Autodesk Inventor part; units mm, degrees
ref_plane "YZ Plane" through (0, 0, 0) normal (1, 0, 0) x (0, 1, 0)
ref_plane "XZ Plane" through (0, 0, 0) normal (0, 1, 0) x (-1, 0, 0)
ref_plane "XY Plane" through (0, 0, 0) normal (0, 0, 1) x (1, 0, 0)
sketch "Sketch5" plane through (0, 0, 0) normal (0, 0, 1) x (1, 0, 0)
  line L0 (0, 0) -> (6.35, 0)
  line L1 (6.35, 0) -> (6.35, 25.4)
  line L2 (6.35, 25.4) -> (0, 25.4)
  line L3 (0, 25.4) -> (0, 0)
  dimension "d21" = 25.4
  dimension "d22" = 6.35
extrude "Extrusion3" add sketch "Sketch5" against normal mid plane 38.1
sketch "Sketch6" plane through (0, 0, 0) normal (0, 0, 1) x (1, 0, 0)
  line L0 (6.35, 25.4) -> (6.35, 0)
  line L1 (0, 25.4) -> (6.35, 25.4)
  line L2 (6.35, 0) -> (0, 0)
  line L3 (0, 0) -> (0, 25.4)
  line L4 (6.35, 0) -> (70.8025, 37.2117)
  line L5 (6.35, 0) -> (80.7733, 0) construction
  line L6 (70.8025, 62.6117) -> (70.8025, 37.2117)
  arc A0 (38.9766, 44.237) -> (62.6234, 57.8895) centre (50.8, 51.0632) ccw
  line L7 (6.35, 25.4) -> (38.9766, 44.237)
  line L8 (62.6234, 57.8895) -> (70.8025, 62.6117)
  dimension "d25" = 30
  dimension "d26" = 27.305
  dimension "d29" = 6.35
  dimension "d30" = 50.8
  dimension "d33" = 0
extrude "Extrusion4" add sketch "Sketch6" along normal mid plane 6.35 contours L7 A0 L8 L6 L4 L0
sketch "Sketch7" plane through (6.35, 0, 19.05) normal (1, 0, 0) x (0, 0, -1)
  line L0 (38.1, 25.4) -> (0, 25.4) construction
  line L1 (6.35, 25.4) -> (6.35, 0) construction
  line L2 (31.75, 25.4) -> (31.75, 0) construction
  line L3 (0, 0) -> (0, 25.4) construction
  line L4 (38.1, 25.4) -> (38.1, 0) construction
  line L5 (0, 0) -> (15.875, 0)
  line L6 (22.225, 0) -> (38.1, 0)
  point P0 (19.05, 0)
  point P1 (6.35, 12.7)
  point P2 (31.75, 12.7)
  dimension "d34" = 6.35
  dimension "d35" = 6.35
sketch "Sketch8" plane through (0, 0, 0) normal (0, 0, 1) x (1, 0, 0)
  line L0 (0, 0) -> (0, 25.4)
  line L1 (6.35, 0) -> (0, 0)
  line L2 (70.8025, 37.2117) -> (6.35, 0)
  line L3 (0, 0) -> (6.35, 0)
  line L4 (0, -3.6662) -> (6.35, 0)
  line L5 (0, 0) -> (0, -3.6662)
extrude "Extrusion5" add sketch "Sketch8" along normal mid plane 38.1
hole "Hole3" at (6.35, 12.7, 12.7) at (6.35, 12.7, -12.7) direction (-1, 0, 0) diameter 3.81 end through all countersink diameter 7.0866 countersink angle 82
sketch "Sketch9" plane through (0, 0, 0) normal (0, 0, 1) x (1, 0, 0)
  line L0 (0, -3.6662) -> (0, 25.4)
  line L1 (0, 25.4) -> (6.35, 25.4)
  line L2 (6.35, 25.4) -> (6.35, 0)
  line L3 (6.35, 25.4) -> (38.9766, 44.237)
  line L4 (6.35, 25.4) -> (0, 25.4)
  line L5 (6.35, 25.4) -> (0, 21.7338)
  line L6 (0, 25.4) -> (0, 21.7338)
  point P0 (0, 0)
extrude "Extrusion6" cut sketch "Sketch9" against normal mid plane 38.1
equation "\"d21\" = supportHeight"
equation "\"d22\" = supportWidth"
equation "\"d23\" = totalScrewHoldWidth"
equation "\"d25\" = supportAngle"
equation "\"d26\" = pipeDiameter"
equation "\"d30\" = distanceFromWallToPipeCenter"
equation "\"d31\" = supportWidth"
equation "\"d47\" = totalScrewHoldWidth"
equation "\"d63\" = totalScrewHoldWidth"
equation "\"pipeDiameter\" = 27.305"
equation "\"distanceFromWallToPipeCenter\" = 50.8"
equation "\"supportHeight\" = 25.4"
equation "\"supportWidth\" = 6.35"
equation "\"screwHoldDepth\" = 6.35"
equation "\"totalScrewHoldWidth\" = 38.1"
equation "\"screwPositionFromTop\" = 6.35"
equation "\"supportAngle\" = 30deg"
properties part number "PipeSupport-2_00-030"
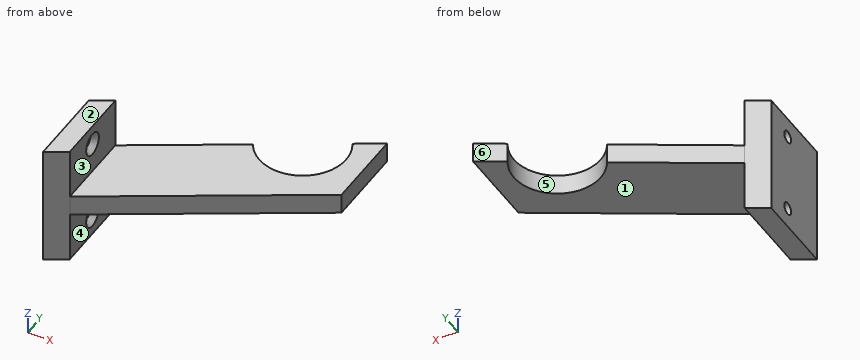
Can you work these out from the model? Positions are in its coordinate system, mm. Face numbers are marked on the shaded views. A direction names the side the tool comes from. Give positions to 0.01 mm unless a question says otherwise; leave off trailing zeros. Order: outer loops, then holes, each group sorted by start corner. A loop starts at its lowest first (then second) coordinate and runs counter-clockwise, first axis right, second up. Notation, with made-up numbers: M 70,44 L 96,44 A17 ccw 96,63 Z; hole C 48.5,45 d1. An arc over 180 degrees is marked long. Use one line per item in the form item = value. Start each with the question number.
Item 1: For the marked faces 1, 2 and 3, which set-ups out of +Z, -Z, +X, -X, +Y, -Y let a thin tool reach every point of the face, with its end or its side?
Item 2: If we section it at B-B (y = 12.7): Write out the boundary of the cut face in (x, z) (3 decimals).
Item 3: We'd pull the mould along X, two halves only. Please class the marked faces 4, 5 and 6: +X half, -X half, draft (parallel to the pull), parting line (faces both ways), or undercut.
Item 4: Will these pins go through, and if not, where does the flat tip stop? pin 1 Ø5 at (y, z) = (17.5, -15) entering from +X; pin 2 Ø4 at (y, z) = (16, -4) entering from +X; pin 3 Ø10 at (x, z) = (40, 4.5) entering from +Y.
Item 5: If we section it at D-D (z = -1.5): Write out the boundary of the cut face in (x, y), then the cut area to 3 significant figures.
Item 6: If I drill on line 1 along Z through (x, y) = (2.1, 12.7) (3 decimals); line 2 along Z through (x, y) = (2, 12); line 3 along Z through (x, y) = (13, 5.5) (3 decimals), over which ranges is the centre line in solid material (lowest first)?
Item 7: If we section it at C-C (y = 1.5): Write out the boundary of the cut face in (x, z) (3 decimals), then the cut area to 3 significant figures.
Item 8: If we section it at A-A (z = -12.7): Write out the boundary of the cut face in (x, y) (3 decimals), then the cut area to 3 significant figures.
Outcome:
q1.face_1 = -Z, +X, +Y, -Y
q1.face_2 = +Z, +X, -X, +Y, -Y
q1.face_3 = +Z, +X, +Y, -Y
q2.outline = M 0,-19.05 L 6.35,-19.05 L 6.35,-16.243 L 4.465,-14.605 L 0,-14.605 Z; M 0,-10.795 L 4.465,-10.795 L 6.35,-9.157 L 6.35,-3.175 L 28.347,-3.175 L 28.347,3.175 L 6.35,3.175 L 6.35,9.157 L 4.465,10.795 L 0,10.795 Z; M 0,14.605 L 4.465,14.605 L 6.35,16.243 L 6.35,19.05 L 0,19.05 Z
q3.face_4 = +X half
q3.face_5 = undercut
q3.face_6 = -X half
q4.pin_1 = 6.35
q4.pin_2 = 37.22
q4.pin_3 = 44.24
q5.outline = M 0,-3.67 L 6.35,0 L 70.8,37.21 L 70.8,62.61 L 62.62,57.89 A13.65 cw 38.98,44.24 L 6.35,25.4 L 0,21.73 Z
q5.area = 1,510 mm2
q6.line_1 = -19.05 to -14.605, -10.795 to 10.795, 14.605 to 19.05
q6.line_2 = -19.05 to -14.47, -10.93 to 10.93, 14.47 to 19.05
q6.line_3 = -3.175 to 3.175
q7.outline = M 0,-19.05 L 6.35,-19.05 L 6.35,-3.175 L 8.948,-3.175 L 8.948,3.175 L 6.35,3.175 L 6.35,19.05 L 0,19.05 Z
q7.area = 258 mm2
q8.outline = M 0,-3.666 L 6.35,0 L 6.35,9.157 L 4.465,10.795 L 0,10.795 Z; M 0,14.605 L 4.465,14.605 L 6.35,16.243 L 6.35,25.4 L 0,21.734 Z
q8.area = 134 mm2
